```python
from build123d import *

# Parameters (mm, degrees)
CROQUIS1_W              = 60
CROQUIS1_H              = 40
SALIENTE_EXTRUIR1_DEPTH = 40
CHAFL_N1_START          = -14.142135624
CHAFL_N1_DEPTH          = 56.568542495


with BuildPart() as part:
    # Croquis1 → Saliente-Extruir1 (new body)
    with BuildSketch(Plane(origin=(0, 0, 0), x_dir=(1, 0, 0), z_dir=(0, 1, 0))):
        Rectangle(CROQUIS1_W, CROQUIS1_H)
    extrude(amount=SALIENTE_EXTRUIR1_DEPTH)

    # Chaflán1: read off the stored shape, not the designer's step
    # Chaflán1 outline → Chaflán1 (cut)
    with BuildSketch(Plane(origin=(0, 0, 0), x_dir=(1, 0, 0), z_dir=(0, 0.7071067811865476, -0.7071067811865476)).offset(CHAFL_N1_START)):
        Polygon((30, -14.849242405), (-9, -42.426406871), (-10, -43.133513652), (-10, -44), (30, -44), align=None)
    extrude(amount=CHAFL_N1_DEPTH, mode=Mode.SUBTRACT)


solid = part.part
```
Part model, mm, in its own coordinate system. Coordinates: 2 decimals unless noted, no trailing zeros. Write each loop counter-clockwise with the first axis right and the second up, starting at its lowest first coordinate (ties: lowest second). Pieces come first, ordered by that corner, then holes.
Item 1: Slice it at B-B (y = 10.5). Write the cut outline in (x, z), and give its area (3 significant figures).
Item 2: Slice it at A-A (z = 7.5). Write the cut outline in (x, y), and give its area (3 significant figures).
Item 3: Probe line 1 (Z direction, x = 9, y = 35); line 2 (Y direction, x = 5.5, z = 11.5); line 3 (X direction, y = 32.5, z = -1.5). List the from-to ranges inside material, lowest first.
Results found:
1. outline: (-30, -20) - (30, -20) - (30, 10.5) - (20.5, 20) - (-30, 20) - close
1. area: 2,350 mm2
2. outline: (-30, 0) - (30, 0) - (30, 13.5) - (3.5, 40) - (-30, 40) - close
2. area: 2,050 mm2
3. line 1: z = -20 to 7
3. line 2: y = 0 to 34
3. line 3: x = -30 to 20
